from build123d import *

# Parameters (mm, degrees)
SKETCH_1_R          = 2.000000000000001
EXTRUDE_1_DEPTH     = 29
SKETCH_2_W          = 20.5
SKETCH_2_H          = 70.28340969233892
EXTRUDE_2_DEPTH     = 3
SKETCH_3_W          = 20.5
SKETCH_3_H          = 7.570852423084727
CUT_EXTRUDE_1_DEPTH = 49.62100286394029
SKETCH_5_R          = 2.5
EXTRUDE_3_DEPTH     = 10
CUT_EXTRUDE_2_REACH = 75.297
SKETCH_8_R          = 1.6000000000000003
SKETCH_9_W          = 20.5
SKETCH_9_H          = 32
CUT_EXTRUDE_3_DEPTH = 65.57298284377197
SKETCH_12_W         = 20.499999999999996
SKETCH_12_H         = 7.57085242308473
SKETCH_12_R         = 2.0000000000000018
SKETCH_12_R_2       = 2.000000000000001
EXTRUDE_5_DEPTH     = 30
EXTRUDE_6_DEPTH     = 10
SKETCH_16_R         = 1.5000000000000004
CUT_EXTRUDE_5_DEPTH = 48.388093987806805
SKETCH_17_R         = 1.5000000000000004
CUT_EXTRUDE_6_DEPTH = 51.404676958704755
EXTRUDE_START       = 10
SKETCH_19_R         = 4
SKETCH_19_R_2       = 2.5000000000000004
EXTRUDE_7_DEPTH     = 10
SKETCH_21_R         = 1.5000000000000004
CUT_EXTRUDE_7_DEPTH = 48.38809406709012
SKETCH_22_R         = 1.5000000000000004
CUT_EXTRUDE_8_DEPTH = 51.404676958704755


with BuildPart() as part:
    # 草图1 → 凸台-拉伸1 (new body)
    # profile 1 of 3: a face of its own
    with BuildSketch(Plane.XY):
        with BuildLine():
            Line((-10.250000000000004, 35.14170484616946), (-10.250000000000004, 20))
            Line((-10.25, 20.000000000000004), (-4.999999999999999, 20.000000000000004))
            Line((-4.999999999999999, 20.000000000000004), (-4.999999999999999, 23.000000000000004))
            ThreePointArc((-5.000000000000001, 23.000000000000004), (-6.414213562373094, 26.4142135623731), (-2.9999999999999982, 25.000000000000004))
            Line((-2.9999999999999982, 25.000000000000004), (3, 25.000000000000004))
            ThreePointArc((3, 25.000000000000004), (5.000000000000001, 27.000000000000004), (7.000000000000002, 25.000000000000004))
            ThreePointArc((7.000000000000002, 25.000000000000004), (6.414213562373095, 23.585786437626908), (4.999999999999999, 23.000000000000004))
            Line((5.000000000000001, 23.000000000000004), (5.000000000000001, 20.000000000000004))
            Line((5, 20.000000000000004), (10.249999999999996, 20.000000000000004))
            Line((10.249999999999996, 20), (10.249999999999996, 35.14170484616946))
            Line((10.249999999999996, 35.14170484616946), (-10.250000000000004, 35.14170484616946))
        make_face()
    # profile 2 of 3: a face of its own
    with BuildSketch(Plane.XY):
        Polygon((10.249999999999996, -20), (-10.25, -20), (-10.250000000000004, -35.14170484616946), (10.249999999999996, -35.14170484616946), align=None)
        with Locations(Location((-4.999999999999999, -25.000000000000004, 0), (0, 0, 180))):
            Circle(SKETCH_1_R, mode=Mode.SUBTRACT)
        with Locations(Location((5.000000000000001, -25.000000000000004, 0), (0, 0, 180))):
            Circle(SKETCH_1_R, mode=Mode.SUBTRACT)
    # profile 3 of 3: a face of its own
    with BuildSketch(Plane.XY):
        with BuildLine():
            Line((-4.999999999999999, 23.000000000000004), (-4.999999999999999, 20.000000000000004))
            Line((-4.999999999999999, 20.000000000000004), (5, 20.000000000000004))
            Line((5.000000000000001, 20.000000000000004), (5.000000000000001, 23.000000000000004))
            ThreePointArc((4.999999999999999, 23.000000000000004), (3.585786437626904, 23.585786437626908), (3, 25.000000000000004))
            Line((3, 25.000000000000004), (-2.9999999999999982, 25.000000000000004))
            ThreePointArc((-2.9999999999999982, 25.000000000000004), (-3.585786437626905, 23.585786437626908), (-5.000000000000001, 23.000000000000004))
        make_face()
    extrude(amount=EXTRUDE_1_DEPTH)

    # 草图2 → 凸台-拉伸2 (add)
    with BuildSketch(Plane.XY.offset(29)):
        Rectangle(SKETCH_2_W, SKETCH_2_H)
    extrude(amount=EXTRUDE_2_DEPTH)

    # 草图3 → 切除-拉伸1 (cut, through all)
    with BuildSketch(Plane(origin=(0, 0, 0), x_dir=(-1, 0, 0), z_dir=(0, 0, -1))):
        with Locations((3.55e-15, -31.356278634627095)):
            Rectangle(SKETCH_3_W, SKETCH_3_H)
        Polygon((-10.249999999999996, 35.14170484616946), (-10.249999999999996, 27.57085242308473), (10.250000000000004, 27.570852423084734), (10.250000000000004, 35.14170484616946), align=None)
    extrude(amount=-CUT_EXTRUDE_1_DEPTH, mode=Mode.SUBTRACT)

    # 草图5 → 凸台-拉伸3 (add)
    with BuildSketch(Plane.XZ.offset(27.570852423084734)):
        with Locations(Location((0, 2.5, 0), (0, 0, 270))):
            Circle(SKETCH_5_R)
    extrude(amount=EXTRUDE_3_DEPTH)

    # 草图8 → 切除-拉伸2 (cut, up to next)
    with BuildSketch(Plane(origin=(0, 27.570852423084734, 0), x_dir=(1, 0, 0), z_dir=(0, 1, 0)), mode=Mode.PRIVATE) as cut_extrude_2_sk1:
        with Locations(Location((1.71e-15, -16.5, 0), (0, 0, 270))):
            Circle(SKETCH_8_R)
    cut_extrude_2_tool1 = extrude(cut_extrude_2_sk1.sketch, amount=-CUT_EXTRUDE_2_REACH, mode=Mode.PRIVATE) & part.part
    # 草图8 → 切除-拉伸2 (cut, up to next)
    with BuildSketch(Plane(origin=(0, 27.570852423084734, 0), x_dir=(1, 0, 0), z_dir=(0, 1, 0)), mode=Mode.PRIVATE) as cut_extrude_2_sk2:
        with Locations(Location((1.22e-15, -26.500000000000004, 0), (0, 0, 270))):
            Circle(SKETCH_8_R)
    cut_extrude_2_tool2 = extrude(cut_extrude_2_sk2.sketch, amount=-CUT_EXTRUDE_2_REACH, mode=Mode.PRIVATE) & part.part
    add(cut_extrude_2_tool1.solids().sort_by_distance((0, 27.570852, 16.5))[0], mode=Mode.SUBTRACT)
    add(cut_extrude_2_tool2.solids().sort_by_distance((0, 27.570852, 26.5))[0], mode=Mode.SUBTRACT)

    # 草图9 → 切除-拉伸3 (cut, through all)
    with BuildSketch(Plane.XZ.offset(27.570852423084734)):
        with Locations((-3.55e-15, 16)):
            Rectangle(SKETCH_9_W, SKETCH_9_H)
    extrude(amount=CUT_EXTRUDE_3_DEPTH, mode=Mode.SUBTRACT)

    # 草图12 → 凸台-拉伸5 (add)
    with BuildSketch(Plane(origin=(0, 0, 0), x_dir=(-1, 0, 0), z_dir=(0, 0, -1))):
        with Locations((1.78e-15, 23.78542621154237)):
            Rectangle(SKETCH_12_W, SKETCH_12_H)
        with Locations((-5.000000000000001, 25.000000000000004)):
            Circle(SKETCH_12_R, mode=Mode.SUBTRACT)
        with Locations((4.999999999999999, 25.000000000000004)):
            Circle(SKETCH_12_R_2, mode=Mode.SUBTRACT)
    extrude(amount=-EXTRUDE_5_DEPTH)

    # 草图13 → 凸台-拉伸6 (add)
    with BuildSketch(Plane(origin=(0, 27.570852423084734, 0), x_dir=(1, 0, 0), z_dir=(0, 1, 0))):
        with BuildLine():
            ThreePointArc((4.456e-14, -7.5), (-2.5, -5.000000000000058), (-7.084e-14, -2.4999999999999996))
            Line((-1.4e-16, -2.4999999999999996), (-5e-17, -1))
            ThreePointArc((7.635e-14, -1), (-3.9999999999999996, -4.999999999999907), (-1.067e-13, -9))
            Line((-4.9e-16, -9), (-4.1e-16, -7.5))
        make_face()
        with BuildLine():
            Line((-5e-17, -1), (-1.4e-16, -2.4999999999999996))
            ThreePointArc((-7.084e-14, -2.4999999999999996), (1.7677669529663447, -3.2322330470336054), (2.500000000000001, -5))
            ThreePointArc((2.500000000000001, -5.000000000000001), (1.767766952966385, -6.767766952966354), (4.456e-14, -7.5))
            Line((-4.1e-16, -7.5), (-4.9e-16, -9))
            ThreePointArc((-1.067e-13, -9), (2.828427124746152, -7.828427124746229), (4.000000000000001, -5.000000000000001))
            ThreePointArc((4.000000000000001, -5), (2.8284271247462174, -2.171572875253837), (7.635e-14, -1))
        make_face()
    extrude(amount=EXTRUDE_6_DEPTH)

    # 草图15 → 旋转1 (revolve)
    with BuildSketch(Plane(origin=(0, 0, 0), x_dir=(0, 0, -1), z_dir=(1, 0, 0))):
        with BuildLine():
            Line((-1, 27.570852423084734), (0, 27.570852423084734))
            ThreePointArc((0, 27.570852423084734), (-0.7128919117369903, 27.930797461014013), (-1, 28.676011694509246))
            Line((-1, 28.676011694509246), (-1, 27.570852423084734))
        make_face()
    revolve(axis=Axis((0, -962.4291475769152, 4.99999999999657), (0, 1, 3.43e-15)))

    # 草图16 → 切除-拉伸5 (cut, through all)
    with BuildSketch(Plane.XY.offset(5)):
        with Locations(Location((4.9e-16, 33.57085242308473, 0), (0, 0, 90))):
            Circle(SKETCH_16_R)
    extrude(amount=-CUT_EXTRUDE_5_DEPTH, mode=Mode.SUBTRACT)

    # 草图17 → 切除-拉伸6 (cut, through all)
    with BuildSketch(Plane(origin=(0, 0, 0), x_dir=(0, 0, -1), z_dir=(1, 0, 0))):
        with Locations((-5, 33.57085242308473)):
            Circle(SKETCH_17_R)
    extrude(amount=-CUT_EXTRUDE_6_DEPTH, mode=Mode.SUBTRACT)

    # 草图19 → 凸台-拉伸7 (add)
    with BuildSketch(Plane.XZ.offset(27.570852423084734).offset(EXTRUDE_START)):
        with Locations(Location((0, 4.999999999999998, 0), (0, 0, 270))):
            Circle(SKETCH_19_R)
        with Locations(Location((0, 4.999999999999998, 0), (0, 0, 90))):
            Circle(SKETCH_19_R_2, mode=Mode.SUBTRACT)
    extrude(amount=-EXTRUDE_7_DEPTH)

    # 草图20 → 旋转2 (revolve)
    with BuildSketch(Plane(origin=(0, 0, 0), x_dir=(0, 0, -1), z_dir=(1, 0, 0))):
        with BuildLine():
            Line((-0.9999999999999983, -27.570852423084734), (0, -27.570852423084734))
            ThreePointArc((0, -27.570852423084734), (-0.7071067811865462, -27.863745641898188), (-0.9999999999999981, -28.570852423084734))
            Line((-0.9999999999999981, -28.570852423084734), (-0.9999999999999983, -27.570852423084734))
        make_face()
    revolve(axis=Axis((0, -1027.5708524230847, 4.999999999996567), (0, 1, 3.43e-15)))

    # 草图21 → 切除-拉伸7 (cut, through all)
    with BuildSketch(Plane.XY.offset(5)):
        with Locations((0, -33.57085242308473)):
            Circle(SKETCH_21_R)
    extrude(amount=-CUT_EXTRUDE_7_DEPTH, mode=Mode.SUBTRACT)

    # 草图22 → 切除-拉伸8 (cut, through all)
    with BuildSketch(Plane(origin=(0, 0, 0), x_dir=(0, 0, -1), z_dir=(1, 0, 0))):
        with Locations((-5, -33.57085242308473)):
            Circle(SKETCH_22_R)
    extrude(amount=-CUT_EXTRUDE_8_DEPTH, mode=Mode.SUBTRACT)


solid = part.part
Geometry check sheet. Reference: the model listing, model coordinates, mm. A direction names the side the tool comes from. Give positions to 0.01 mm unless a question says otherwise; leave off trailing zeros. Order: outer loops, then holes, each group sorted by start corner. A loop starts at its lowest first (then second) coordinate and runs counter-clockwise, first axis right, second up. Notation, with made-up numbers: (87, 20.5) - (98, 20.5) arc R24 cw to (98, 59.5) - close; hole circle Ø8 at (70.25, 30.5). An arc over 180 degrees is marked (long way). Use one line per item in the form item = value.
1) Sectioned sample at D-D (y = -17). Record the boundary of the cut face in (x, z).
Working result:
outline = (-10.25, 29) - (10.25, 29) - (10.25, 32) - (-10.25, 32) - close
2) Sectioned sample at A-A (z = 13.5). Record the boundary of the cut face in (x, y), and give its area (3 significant figures).
Working result:
outline = (-10.25, -27.57) - (10.25, -27.57) - (10.25, -20) - (-10.25, -20) - close; (-10.25, 20) - (10.25, 20) - (10.25, 27.57) - (-10.25, 27.57) - close; hole circle Ø4 at (-5, -25); hole circle Ø4 at (-5, 25); hole circle Ø4 at (5, -25); hole circle Ø4 at (5, 25)
area = 260 mm^2
3) Material ranges on probe 1 along Y at (x, z) = (-5.25, 8.5); probe 2 along Y at (x, z) = (8.5, 21.5); probe 3 along X at (y, z) = (-25, 15), recorded low to high. Write a range as from..to.
Working result:
probe_1 = -27.57..-26.98, -23.02..-20, 20..23.02, 26.98..27.57
probe_2 = -27.57..-20, 20..27.57
probe_3 = -10.25..-7, -3..3, 7..10.25
4) Sectioned sample at B-B (z = 5). Count the separate pieces of the cut face and the enclosed holes in it, and give its area (3 significant figures).
Working result:
separate_pieces = 4
enclosed_holes = 4
area = 312 mm^2
5) Access from +Z, -Z, +X, -X, +Y, -Y to the whole of each face (thin tool, end or side, straight path). Record for faces 1 (the face through (1.69, 32.5, 6.84)), 2 (the face through (2.22, -32.64, 6.15)), 3 (the face through (5, 25, 29)), 4 (the face through (0, 20, 14)).
Working result:
face_1 = +Y
face_2 = -Y
face_3 = -Z
face_4 = -Z, +X, -X
6) Draft check along Z on faces 5 (the face through (-2.99, 34.02, 3.57)), 6 (the face through (0, 24, 0)), 7 (the face through (0, -20, 14)). Enter one of: released by +Z, released by -Z, zero draft, split by the parting line, or undercut.
Working result:
face_5 = undercut
face_6 = released by -Z
face_7 = zero draft
7) Sectioned sample at C-C (y = -25). Record the boundary of the cut face in (x, z), and give its area (3 significant figures).
Working result:
outline = (-10.25, 0) - (-7, 0) - (-7, 29) - (-3, 29) - (-3, 0) - (3, 0) - (3, 29) - (7, 29) - (7, 0) - (10.25, 0) - (10.25, 32) - (-10.25, 32) - close
area = 424 mm^2
8) Depth check by flat-ended pin: pin 1 Ø4 at (x, z) = (0.5, 6) entering from -Y; pin 2 Ø10 at (x, z) = (3, 19.5) entering from -Y; pin 3 Ø5 at (x, z) = (3.5, 28.5) entering from +Y; pin 4 Ø3 at (x, y) = (5, -25) entering from -Z. Enter the tip coordinate at first touch or a pass-through.
Working result:
pin_1 = -37.57
pin_2 = -27.57
pin_3 = 27.57
pin_4 = 29
